Could you check a few things on this model? Use its own coordinates, in mm. A direction names the side the tool comes from. Give positions to 0.01 mm unless a question says otherwise; leave off trailing zeros. Loops run counter-clockwise (first coordinate to the right, second up) from the corner with the lowest first, then second, coordinate; pieces in that order, holes last.
1. I need wall thicknesses on line 1 along X through (y, z) = (19.5, 0); line 2 along X through (y, z) = (76.5, 0). Which ranges of each line are inside material? Lowest first, please.
2. Imagine slicing it at C-C (y = 117). List the corners of the cut face in (x, z) for me, plus the area to 3 significant figures.
3. Imagine slicing it at A-A (z = 0). List the corners of the cut face in (x, y) for me, plus the area to 3 significant figures.
4. Imagine slicing it at B-B (x = 0). List the corners of the cut face in (y, z) for me, plus the area to 3 significant figures.
5. For P1, Ø1, axis at y = 23.5, z = -88, coming from the +X side; P2, Ø1.5, axis at x = -96.5, y = 103, coming from the -Z side; P3, Ø2, axis at x = -115.5, y = 151.5, coming from the -Z side, each with a flat end and sliding along its axis, tell me the tip position at first contact or that it passes through.
6. For faces 1 (the flat face through (2, 0, 36)), 2 (the flat face through (-29, 6, -2)), which set-ups out of +Z, -Z, +X, -X, +Y, -Y let a thin tool reach every point of the face, with its end or its side?
7. Imagine slicing it at D-D (z = 128.5). List the corners of the cut face in (x, y) for me.
```python
from build123d import *

# Parameters (mm, degrees)
FLOOR_SKETCH_R          = 175
FLOOR_SKETCH_R_2        = 12.5
FLOOR_TANK_LID_DEPTH    = 6
BASKET_LEDGE_SKETCH_R   = 152
BASKET_LEDGE_SKETCH_R_2 = 140
BASKET_LEDGE_DEPTH      = 31
HOUSING_WALL_SKETCH_R   = 155
HOUSING_WALL_SKETCH_R_2 = 151
HOUSING_WALL_DEPTH      = 210


with BuildPart() as part:
    # Floor Sketch → Floor - Tank Lid (new body)
    with BuildSketch(Plane(origin=(0, 0, 0), x_dir=(1, 0, 0), z_dir=(0, 1, 0))):
        with Locations(Location((0, 0, 0), (0, 0, 270))):
            Circle(FLOOR_SKETCH_R)
        with Locations(Location((0, 0, 0), (0, 0, 270))):
            Circle(FLOOR_SKETCH_R_2, mode=Mode.SUBTRACT)
    extrude(amount=FLOOR_TANK_LID_DEPTH)

    # Basket Ledge Sketch → Basket Ledge (add)
    with BuildSketch(Plane(origin=(0, 0, 0), x_dir=(1, 0, 0), z_dir=(0, 1, 0))):
        with Locations(Location((0, 0, 0), (0, 0, 270))):
            Circle(BASKET_LEDGE_SKETCH_R)
        with Locations(Location((0, 0, 0), (0, 0, 270))):
            Circle(BASKET_LEDGE_SKETCH_R_2, mode=Mode.SUBTRACT)
    extrude(amount=BASKET_LEDGE_DEPTH)

    # Housing Wall Sketch → Housing Wall (add)
    with BuildSketch(Plane(origin=(0, 0, 0), x_dir=(1, 0, 0), z_dir=(0, 1, 0))):
        with Locations(Location((0, 0, 0), (0, 0, 270))):
            Circle(HOUSING_WALL_SKETCH_R)
        with Locations(Location((0, 0, 0), (0, 0, 270))):
            Circle(HOUSING_WALL_SKETCH_R_2, mode=Mode.SUBTRACT)
    extrude(amount=HOUSING_WALL_DEPTH)


solid = part.part
```
Derived:
1. line 1: x = -155 to -140, 140 to 155
1. line 2: x = -155 to -151, 151 to 155
2. outline: circle Ø310 at (0, 0); hole circle Ø302 at (0, 0)
2. area: 3,850 mm2
3. outline: (-175, 0) - (-12.5, 0) - (-12.5, 6) - (-140, 6) - (-140, 31) - (-151, 31) - (-151, 210) - (-155, 210) - (-155, 6) - (-175, 6) - close; (12.5, 0) - (175, 0) - (175, 6) - (155, 6) - (155, 210) - (151, 210) - (151, 31) - (140, 31) - (140, 6) - (12.5, 6) - close
3. area: 4,130 mm2
4. outline: (0, -175) - (6, -175) - (6, -155) - (210, -155) - (210, -151) - (31, -151) - (31, -140) - (6, -140) - (6, -12.5) - (0, -12.5) - close; (0, 12.5) - (6, 12.5) - (6, 140) - (31, 140) - (31, 151) - (210, 151) - (210, 155) - (6, 155) - (6, 175) - (0, 175) - close
4. area: 4,130 mm2
5. P1: stops at x = 127.94
5. P2: stops at z = -121.89
5. P3: stops at z = -104.47
6. face 1: +Z, -Z, +X, -X, -Y
6. face 2: +Y
7. outline: (-118.8, 0) - (118.8, 0) - (118.8, 6) - (86.68, 6) - (86.68, 210) - (79.3, 210) - (79.3, 31) - (55.57, 31) - (55.57, 6) - (-55.57, 6) - (-55.57, 31) - (-79.3, 31) - (-79.3, 210) - (-86.68, 210) - (-86.68, 6) - (-118.8, 6) - close
